Part model, mm, in its own coordinate system. A direction names the side the tool comes from. Round coordinates to 2 decimals unless told otherwise and drop trailing zeros. Write each loop counter-clockwise with the first axis right and the second up, starting at its lowest first coordinate (ties: lowest second). Pieces come first, ordered by that corner, then holes.
1) Saw through at A-A on y = -23.5. Write the cut outline in (x, z), and give its area (3 significant figures).
2) Flat gauge pins, fed straight in: pin 1 (0.8 mm diameter, centred on x = 28.5, y = -1, fed in from +Z); pin 2 (8 mm diameter, centred on x = 19.5, z = 0.5, fed in from -Y); pin 3 (0.8 mm diameter, centred on x = 0, y = 19, fed in from +Z); pin 4 (2 mm diameter, centred on x = 4.5, z = 7, fed in from -Y). Where does each tip first touch, or does it go through?
3) Which spindle directions (+Z, -Z, +X, -X, +Y, -Y) get a long thin tool onto all of the face, cutting with end or side? Do faces 4 (the flat face through (-6.88, 15.232, 7.936)), 5 (the flat face through (-8, -14, 8)), 6 (the cylindrical face through (8.57, 20.95, 5.56)), 7 (the flat face through (5, 17, 1)). Say none if no direction does.
4) Pull direction Z, two halves, no side cores. Call faces 1 (the cylindrical face through (-9.45, 27.07, -1.15)), 2 (the flat face through (8.3, 15, 5)), 3 (the flat face through (-4.08, 15.232, 7.914)): +Z half, -Z half, draft (parallel to the pull), parting line (faces both ways), or undercut.
5) Saw through at D-D on y = 0. Write the cut outline in (x, z).
6) Drill centre lines: L1, parallel to Y at x = 12.5, z = -4; L2, parallel to Y at x = 0, z = 7; L3, parallel to X at y = 25, z = -9.25. Where is each one in solid material? Low to high.
7) Saw through at C-C on y = -8. Write the cut outline in (x, z).
8) Saw through at B-B on x = 12.5. Write the cut outline in (y, z).
```python
from build123d import *

# Parameters (mm, degrees)
SKETCH_R             = 1.65
SKETCH_W             = 7
SKETCH_H             = 2
PAD_DEPTH            = 27.5
SKETCH001_R          = 1.65
POCKET_DEPTH         = 12.001
POCKET_DEPTH_BACK    = -10.001
SKETCH002_R          = 6.3
POCKET001_DEPTH      = 6.5
SKETCH003_W          = 7
SKETCH003_H          = 28
POCKET002_DEPTH      = 10
SKETCH004_W          = 18
SKETCH004_H          = 1
POCKET003_DEPTH      = 1
POCKET004_DEPTH      = 2.5
POCKET005_DEPTH      = 2.5
SKETCH007_W          = 18
SKETCH007_H          = 7
SKETCH007_H_2        = 7.5
POCKET006_DEPTH      = 22.001
SKETCH008_R          = 1.25
POCKET007_DEPTH      = 12.001
POCKET007_DEPTH_BACK = -10.001
FILLET_R             = 1.5


with BuildPart() as part:
    # Sketch → Pad (new body, symmetric)
    with BuildSketch(Plane.XZ):
        with BuildLine():
            ThreePointArc((-27.325971, 6), (-22.5, -7.7), (-17.674029, 6))
            Line((-17.674029, 6), (-17.674029, 10))
            Line((-17.674029, 10), (17.674029, 10))
            Line((17.674029, 10), (17.674029, 6))
            ThreePointArc((17.674029, 6), (22.5, -7.7), (27.325971, 6))
            Line((29.825971, 6), (27.325971, 6))
            Line((32.5, 2.181091), (29.825971, 6))
            Line((32.5, -12), (32.5, 2.181091))
            Line((-32.5, -12), (32.5, -12))
            Line((-32.5, 2.181091), (-32.5, -12))
            Line((-29.825971, 6), (-32.5, 2.181091))
            Line((-27.325971, 6), (-29.825971, 6))
        make_face()
        with Locations((-5.5, 5.5)):
            Circle(SKETCH_R, mode=Mode.SUBTRACT)
        with Locations((5.5, 5.5)):
            Circle(SKETCH_R, mode=Mode.SUBTRACT)
        with Locations((-5.5, 0)):
            Rectangle(SKETCH_W, SKETCH_H, mode=Mode.SUBTRACT)
        with Locations((5.5, 0)):
            Rectangle(SKETCH_W, SKETCH_H, mode=Mode.SUBTRACT)
    extrude(amount=PAD_DEPTH, both=True)

    # Sketch001 → Pocket (cut, two sides)
    with BuildSketch(Plane.XY) as pocket_sk:
        with Locations((-12.5, 17.5)):
            Circle(SKETCH001_R)
        with Locations((12.5, 17.5)):
            Circle(SKETCH001_R)
        with Locations((-12.5, -17.5)):
            Circle(SKETCH001_R)
        with Locations((12.5, -17.5)):
            Circle(SKETCH001_R)
        with Locations((0, 17.5)):
            Circle(SKETCH001_R)
        with Locations((0, -17.5)):
            Circle(SKETCH001_R)
    extrude(amount=-POCKET_DEPTH, mode=Mode.SUBTRACT)
    extrude(pocket_sk.sketch, amount=-POCKET_DEPTH_BACK, mode=Mode.SUBTRACT)

    # Sketch002 (on DatumPlane) → Pocket001 (cut)
    with BuildSketch(Plane.XY.offset(-11)):
        with Locations((-8, 8)):
            Circle(SKETCH002_R)
        with Locations((8, 8)):
            Circle(SKETCH002_R)
        with Locations((8, -8)):
            Circle(SKETCH002_R)
        with Locations((-8, -8)):
            Circle(SKETCH002_R)
    extrude(amount=POCKET001_DEPTH, mode=Mode.SUBTRACT)

    # Sketch003 (on DatumPlane) → Pocket002 (cut)
    with BuildSketch(Plane.XY.offset(10)):
        with Locations((-5.5, 0)):
            Rectangle(SKETCH003_W, SKETCH003_H)
        with Locations((5.5, 0)):
            Rectangle(SKETCH003_W, SKETCH003_H)
    extrude(amount=-POCKET002_DEPTH, mode=Mode.SUBTRACT)

    # Sketch004 (on DatumPlane) → Pocket003 (cut)
    with BuildSketch(Plane.XY.offset(10)):
        with Locations((0, 15)):
            Rectangle(SKETCH004_W, SKETCH004_H)
        with Locations((0, 17)):
            Rectangle(SKETCH004_W, SKETCH004_H)
        with Locations((0, 19)):
            Rectangle(SKETCH004_W, SKETCH004_H)
        with Locations((0, 21)):
            Rectangle(SKETCH004_W, SKETCH004_H)
        with Locations((0, 23)):
            Rectangle(SKETCH004_W, SKETCH004_H)
        with Locations((0, 25)):
            Rectangle(SKETCH004_W, SKETCH004_H)
        with Locations((0, 27)):
            Rectangle(SKETCH004_W, SKETCH004_H)
        with Locations((0, -27)):
            Rectangle(SKETCH004_W, SKETCH004_H)
        with Locations((0, -25)):
            Rectangle(SKETCH004_W, SKETCH004_H)
        with Locations((0, -23)):
            Rectangle(SKETCH004_W, SKETCH004_H)
        with Locations((0, -21)):
            Rectangle(SKETCH004_W, SKETCH004_H)
        with Locations((0, -19)):
            Rectangle(SKETCH004_W, SKETCH004_H)
        with Locations((0, -17)):
            Rectangle(SKETCH004_W, SKETCH004_H)
        with Locations((0, -15)):
            Rectangle(SKETCH004_W, SKETCH004_H)
    extrude(amount=-POCKET003_DEPTH, mode=Mode.SUBTRACT)

    # Sketch005 (on DatumPlane) → Pocket004 (cut)
    with BuildSketch(Plane.XZ.offset(14)):
        Polygon((-5.5, 2.266838), (-2.7, 3.883419), (-2.7, 7.116581), (-5.5, 8.733162), (-8.3, 7.116581), (-8.3, 3.883419), align=None)
        Polygon((8.3, 3.883419), (8.3, 7.116581), (5.5, 8.733162), (2.7, 7.116581), (2.7, 3.883419), (5.5, 2.266838), align=None)
    extrude(amount=POCKET004_DEPTH, mode=Mode.SUBTRACT)

    # Sketch006 (on DatumPlane) → Pocket005 (cut)
    with BuildSketch(Plane.XZ.offset(-14)):
        Polygon((-2.7, 3.883419), (-2.7, 7.116581), (-5.5, 8.733162), (-8.3, 7.116581), (-8.3, 3.883419), (-5.5, 2.266838), align=None)
        Polygon((8.3, 3.883419), (8.3, 7.116581), (5.5, 8.733162), (2.7, 7.116581), (2.7, 3.883419), (5.5, 2.266838), align=None)
    extrude(amount=-POCKET005_DEPTH, mode=Mode.SUBTRACT)

    # Sketch007 (on DatumPlane) → Pocket006 (cut, through all)
    with BuildSketch(Plane.XY.offset(10)):
        with Locations((0, 24)):
            Rectangle(SKETCH007_W, SKETCH007_H)
        with Locations((0, -23.75)):
            Rectangle(SKETCH007_W, SKETCH007_H_2)
    extrude(amount=-POCKET006_DEPTH, mode=Mode.SUBTRACT)

    # Sketch008 → Pocket007 (cut, two sides)
    with BuildSketch(Plane.XY) as pocket007_sk:
        Circle(SKETCH008_R)
    extrude(amount=-POCKET007_DEPTH, mode=Mode.SUBTRACT)
    extrude(pocket007_sk.sketch, amount=-POCKET007_DEPTH_BACK, mode=Mode.SUBTRACT)

    # Fillet
    fillet_edges = [part.edges().sort_by_distance(p)[0] for p in [
        (-9, -20, 5.5),
        (-9, -20, -6.5),
        (9, -20, 5.5),
        (9, -20, -6.5),
        (-9, -27.5, -1),
        (9, -27.5, -1),
        (9, 20.5, 5.5),
        (9, 20.5, -6.5),
        (9, 27.5, -1),
        (-9, 20.5, 5.5),
        (-9, 20.5, -6.5),
        (-9, 27.5, -1),
        (32.5, 27.5, -4.909454),
        (-32.5, 27.5, -4.909454),
        (-32.5, -27.5, -4.909454),
        (32.5, -27.5, -4.909454),
    ]]
    fillet(fillet_edges, radius=FILLET_R)


solid = part.part
```
Completed:
1. outline: (-32.5, -12) - (-9, -12) - (-9, 10) - (-17.67, 10) - (-17.67, 6) arc R7.7 cw (long way) to (-27.33, 6) - (-29.83, 6) - (-32.5, 2.18) - close; (9, -12) - (32.5, -12) - (32.5, 2.18) - (29.83, 6) - (27.33, 6) arc R7.7 cw (long way) to (17.67, 6) - (17.67, 10) - (9, 10) - close
1. area: 555 mm2
2. pin 1: stops at z = 6
2. pin 2: passes through
2. pin 3: stops at z = 9
2. pin 4: stops at y = -20
3. face 4: none
3. face 5: +Z
3. face 6: +Z, -Z, +Y
3. face 7: +Y, -Y
4. face 1: draft
4. face 2: undercut
4. face 3: undercut
5. outline: (-32.5, -12) - (-1.25, -12) - (-1.25, 10) - (-2, 10) - (-2, -1) - (-9, -1) - (-9, 10) - (-17.67, 10) - (-17.67, 6) arc R7.7 cw (long way) to (-27.33, 6) - (-29.83, 6) - (-32.5, 2.18) - close; (1.25, -12) - (32.5, -12) - (32.5, 2.18) - (29.83, 6) - (27.33, 6) arc R7.7 cw (long way) to (17.67, 6) - (17.67, 10) - (9, 10) - (9, -1) - (2, -1) - (2, 10) - (1.25, 10) - close
6. L1: y = -27.5 to -19.15, -15.85 to 15.85, 19.15 to 27.5
6. L2: y = -20 to -19.15, -15.85 to -1.25, 1.25 to 15.85, 19.15 to 20.5
6. L3: x = -32.5 to -9, 9 to 32.5
7. outline: (-32.5, -12) - (32.5, -12) - (32.5, 2.18) - (29.83, 6) - (27.33, 6) arc R7.7 cw (long way) to (17.67, 6) - (17.67, 10) - (9, 10) - (9, -1) - (2, -1) - (2, 10) - (-2, 10) - (-2, -1) - (-9, -1) - (-9, 10) - (-17.67, 10) - (-17.67, 6) arc R7.7 cw (long way) to (-27.33, 6) - (-29.83, 6) - (-32.5, 2.18) - close; hole (-14.3, -11) - (-1.7, -11) - (-1.7, -4.5) - (-14.3, -4.5) - close; hole (1.7, -11) - (14.3, -11) - (14.3, -4.5) - (1.7, -4.5) - close
8. outline: (-27.5, -12) - (-19.15, -12) - (-19.15, 10) - (-27.5, 10) - close; (-15.85, -12) - (15.85, -12) - (15.85, 10) - (-15.85, 10) - close; (19.15, -12) - (27.5, -12) - (27.5, 10) - (19.15, 10) - close; hole (-12.41, -11) - (-3.59, -11) - (-3.59, -4.5) - (-12.41, -4.5) - close; hole (3.59, -11) - (12.41, -11) - (12.41, -4.5) - (3.59, -4.5) - close
